Source: three-view drawing plus pictorial views. Frame: mm from the lowest corner of the part. Coordinates: 2 decimals unless noted, no trailing zeros. Loops run counter-clockwise (first coordinate to the right, second up) from the corner with the lowest first, then second, coordinate; pieces in that order, holes last. Notation, with made-up numbers: M 35.25,21 L 45.25,21 A29 ccw 45.25,54 Z; hole C 6,44 d7. An arc over 180 degrees is marked long. Use a Markdown table: item, result. Add a question column.
1. Section C-C on x = 577.5. Output: boundary loops of the cut face in (y, z), then the cut area to 3 significant figures.
2. Section D-D on y = 66.5. Output: boundary loops of the cut face in (x, z), then the cut area to 3 significant figures.
3. Line query: L1, parallel to Z at x = 207, y = 122.5; L2, parallel to X at y = 93, z = 734; L3, parallel to Z at x = 246, y = 112.5. Output: solid intervals per line, ascending. Write a range as [from, to].
4. Section B-B on y = 112. Output: boundary loops of the cut face in (x, z).
5. Section A-A on z = 373. Output: boundary loops of the cut face in (x, y), then the cut area to 3 significant figures.
6. Pin query (flat end, axial travel): pin 1 (6 mm diameter, centred on x = 103, z = 770.5, fed in from -Y); pin 2 (15 mm diameter, centred on y = 16.5, z = 175.5, fed in from -X). Return the tip coordinate at first contact, or that it passes through.
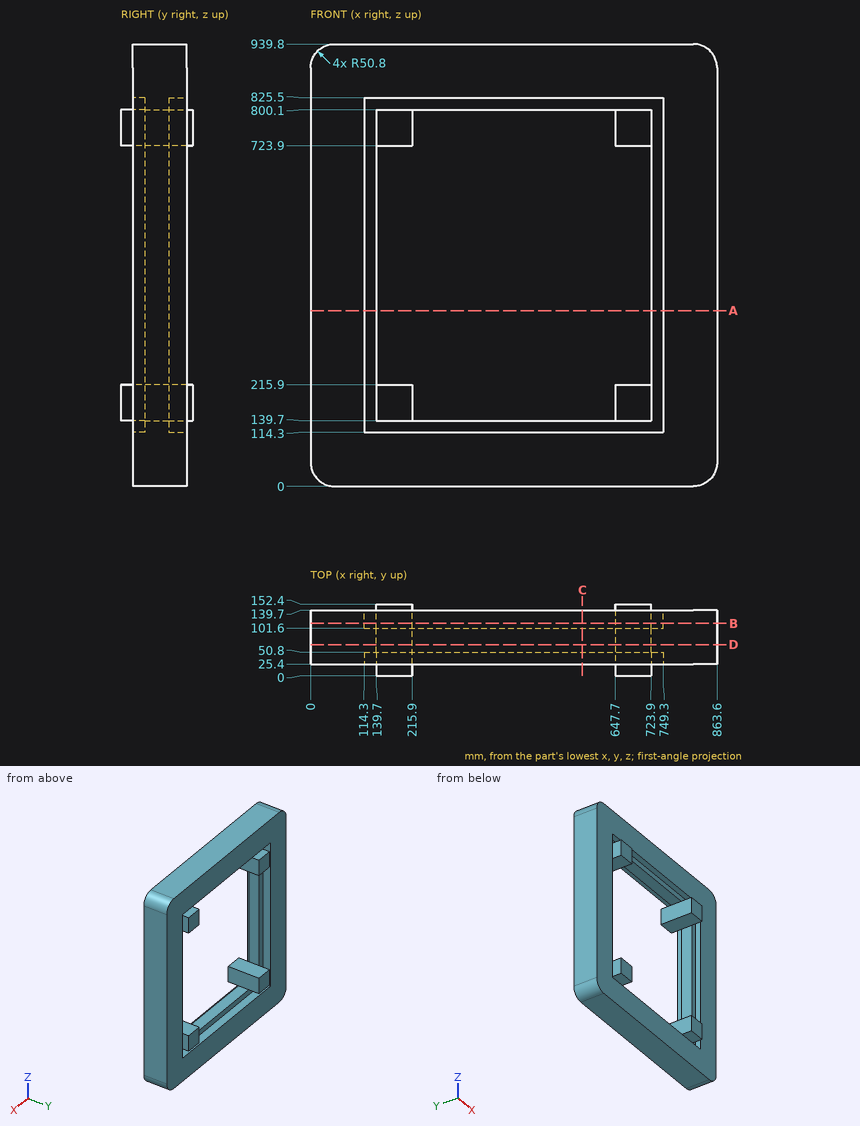
Answers below:
| question | item | result |
|---|---|---|
| 1 | outline | M 25.4,0 L 139.7,0 L 139.7,114.3 L 101.6,114.3 L 101.6,139.7 L 50.8,139.7 L 50.8,114.3 L 25.4,114.3 Z; M 25.4,825.5 L 50.8,825.5 L 50.8,800.1 L 101.6,800.1 L 101.6,825.5 L 139.7,825.5 L 139.7,939.8 L 25.4,939.8 Z |
| 1 | area | 28,700 mm² |
| 2 | outline | M 0,50.8 A50.8 ccw 50.8,0 L 812.8,0 A50.8 ccw 863.6,50.8 L 863.6,889 A50.8 ccw 812.8,939.8 L 50.8,939.8 A50.8 ccw 0,889 Z; hole M 139.7,215.9 L 215.9,215.9 L 215.9,139.7 L 647.7,139.7 L 647.7,215.9 L 723.9,215.9 L 723.9,723.9 L 647.7,723.9 L 647.7,800.1 L 215.9,800.1 L 215.9,723.9 L 139.7,723.9 Z |
| 2 | area | 447,000 mm² |
| 3 | L1 | z = [0, 114.3], [139.7, 215.9], [723.9, 800.1], [825.5, 939.8] |
| 3 | L2 | x = [0, 215.9], [647.7, 863.6] |
| 3 | L3 | z = [0, 114.3], [825.5, 939.8] |
| 4 | outline | M 0,50.8 A50.8 ccw 50.8,0 L 812.8,0 A50.8 ccw 863.6,50.8 L 863.6,889 A50.8 ccw 812.8,939.8 L 50.8,939.8 A50.8 ccw 0,889 Z; M 139.7,139.7 L 215.9,139.7 L 215.9,215.9 L 139.7,215.9 Z; M 139.7,723.9 L 215.9,723.9 L 215.9,800.1 L 139.7,800.1 Z; M 647.7,139.7 L 723.9,139.7 L 723.9,215.9 L 647.7,215.9 Z; M 647.7,723.9 L 723.9,723.9 L 723.9,800.1 L 647.7,800.1 Z; hole M 114.3,114.3 L 749.3,114.3 L 749.3,825.5 L 114.3,825.5 Z |
| 5 | outline | M 0,25.4 L 114.3,25.4 L 114.3,50.8 L 139.7,50.8 L 139.7,101.6 L 114.3,101.6 L 114.3,139.7 L 0,139.7 Z; M 723.9,50.8 L 749.3,50.8 L 749.3,25.4 L 863.6,25.4 L 863.6,139.7 L 749.3,139.7 L 749.3,101.6 L 723.9,101.6 Z |
| 5 | area | 28,700 mm² |
| 6 | pin 1 | stops at y = 25.4 |
| 6 | pin 2 | stops at x = 139.7 |
